Design review of the part shown in the three views and the two pictorial views. Dimensions are in mm from the part's minimum x, y and z. Round coordinates to 2 decimals unless told otherwise and drop trailing zeros. Loops run counter-clockwise (first coordinate to the right, second up) from the corner with the lowest first, then second, coordinate; pieces in that order, holes last. Notation, with made-up numbers: M -16.5,29.25 L -3.5,29.25 A25 cw -3.5,43.25 Z; hole C -40,58.5 d6. An arc over 180 degrees is marked long. Return JSON: item names as keys, results as strings. Group by question number.
Q1. Clearance check with a flat-ended pin moving along its axis: pin 1 Ø18.5 at (x, z) = (42.5, 72.31) entering from -Y. State where the tip first meets the part, or that it passes through.
Q2. Consider section C-C (x = 142). State the section outline as (y, z) points.
Q3. Consider section A-A (x = 24). State the section outline as (y, z) points.
Q4. Consider section B-B (y = 1.85). State the section outline as (x, z) points (1 decimal), and give its area (3 significant figures).
Q5. To check wall thickness, follow line 1 along X through (y, z) = (0.65, 163) (1 decimal); line 2 along Z through (x, y) = (108.5, 1.95); line 3 along Z through (x, y) = (47, 2.95) (1 decimal). State the ranges of each line that lie inside material, in increasing order.
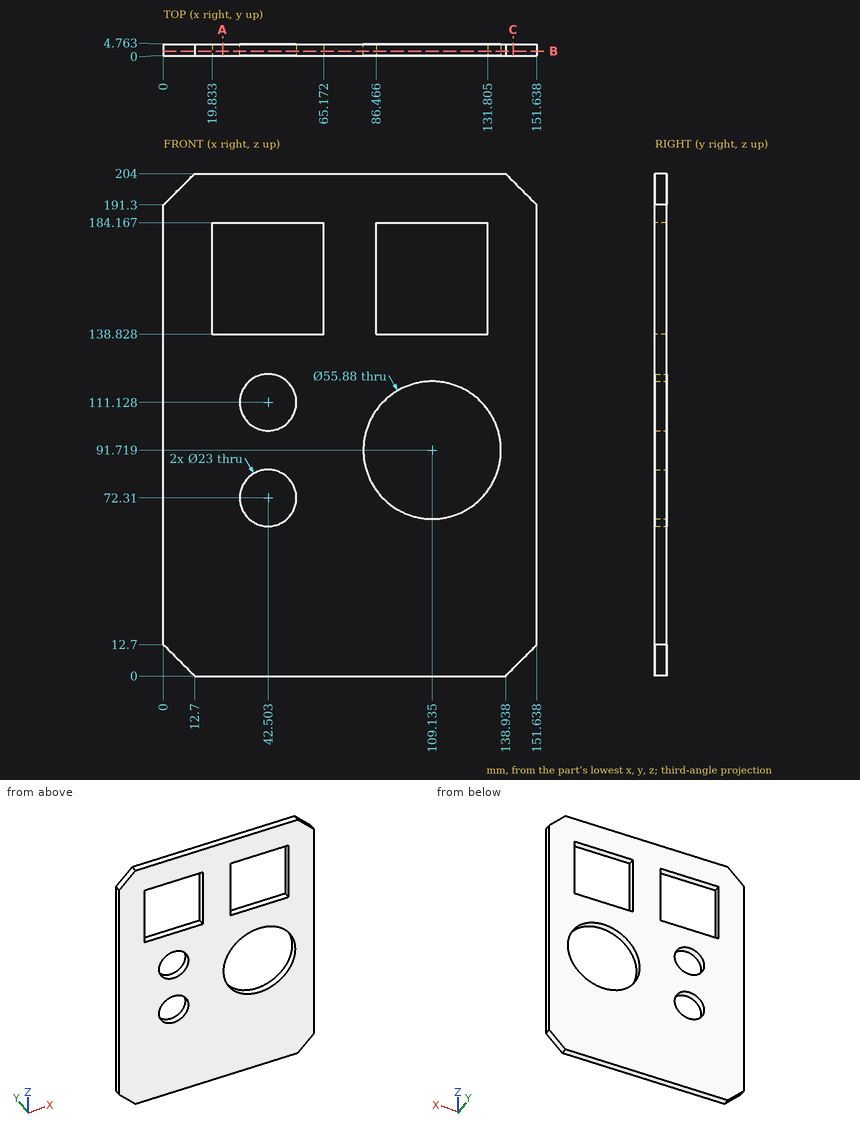
Values:
{
 "1": {"pin 1": "passes through"},
 "2": {"outline": "M 0,3.06 L 4.76,3.06 L 4.76,200.94 L 0,200.94 Z"},
 "3": {"outline": "M 0,0 L 4.76,0 L 4.76,138.83 L 0,138.83 Z; M 0,184.17 L 4.76,184.17 L 4.76,204 L 0,204 Z"},
 "4": {"outline": "M 0,12.7 L 12.7,0 L 138.9,0 L 151.6,12.7 L 151.6,191.3 L 138.9,204 L 12.7,204 L 0,191.3 Z; hole M 19.8,138.8 L 65.2,138.8 L 65.2,184.2 L 19.8,184.2 Z; hole C 42.5,72.3 d23; hole C 42.5,111.1 d23; hole C 109.1,91.7 d55.9; hole M 86.5,138.8 L 131.8,138.8 L 131.8,184.2 L 86.5,184.2 Z", "area": "23,200 mm2"},
 "5": {"line 1": "x = 0 to 19.8, 65.2 to 86.5, 131.8 to 151.6", "line 2": "z = 0 to 63.79, 119.65 to 138.83, 184.17 to 204", "line 3": "z = 0 to 61.7, 82.9 to 100.5, 121.7 to 138.8, 184.2 to 204"}
}
